The model under review builds one solid part; all positions refer to its coordinate system, in mm. A direction names the side the tool comes from. Coordinates: 2 decimals unless noted, no trailing zeros. Loops run counter-clockwise (first coordinate to the right, second up) from the corner with the lowest first, then second, coordinate; pieces in that order, holes last. Notation, with made-up numbers: M 45,25 L 82,25 A26 cw 82,59 Z; hole C 87.25,-20.5 d7. An arc over 180 degrees is marked long. Use one line per item in the form item = value.
Solid Edge part; units mm, degrees
sketch "Sketch1" plane through (0, 0, 0) normal (0, 0, 1) x (1, 0, 0)
  circle A0 centre (0, 0) radius 7.1374
extrude "Protrusion1" add sketch "Sketch1" along normal blind 6.35
sketch "Sketch2" plane through (0, 0, 0) normal (0, 0, -1) x (0, 1, 0)
  circle A0 centre (0, 0) radius 4.7625
extrude "Protrusion2" add sketch "Sketch2" along normal blind 12.7
sketch "Sketch3" plane through (0, 0, -12.7) normal (0, 0, -1) x (0, 1, 0)
  circle A0 centre (0, 0) radius 3.9688
extrude "Protrusion3" add sketch "Sketch3" along normal blind 12.7
sketch "Sketch4" plane through (0, 0, 6.35) normal (0, 0, 1) x (0, 1, 0)
  line L0 (-2.3876, 1.3131) -> (0, 2.8792)
  line L1 (-2.3876, -1.5424) -> (-2.3876, 1.3131)
  line L2 (-2.3876, -1.5424) -> (0, -2.8792)
  line L3 (2.3876, -1.5424) -> (0, -2.8792)
  line L4 (2.3876, -1.5424) -> (2.3876, 1.3131)
  line L5 (2.3876, 1.3131) -> (0, 2.8792)
extrude "Cutout1" cut sketch "Sketch4" against normal blind 3.175
chamfer "Chamfer1" distance 0.7874 angle 45 1 edges at (0, -3.9688, -25.4)
properties part number "24103079"
1. Machinability: for faces 1 (the face through (0, -3, 6.35)), 2 (the face through (2.2, 1.21, 4.78)), 3 (the face through (2.9, -3.78, -6.26)), which of the approach directions +Z, -Z, +X, -X, +Y, -Y give a long, thin tool a straight path to every point of the face, cutting with its end or side? Answer none if there is none.
Response values:
face_1 = +Z, +X, -X, +Y, -Y
face_2 = +Z
face_3 = -Z
2. Add section B-B (z = -5). State the section outline as (x, y) points (1 decimal).
Response values:
outline = C 0,0 d9.5
3. Add section D-D (z = -16.5). State the section outline as (x, y) points.
Response values:
outline = C 0,0 d7.94
4. Add section C-C (y = -5.25). State the section outline as (x, z) points.
Response values:
outline = M -4.84,0 L 4.84,0 L 4.84,6.35 L -4.84,6.35 Z
5. Insertion check: P1, Ø4, axis at x = 4.5, z = 1, coming from the +Y side; P2, Ø1, axis at x = 5, y = 2, coming from the -Z side; P3, Ø2, axis at y = 3, z = -13, coming from the -X side. Each pin has a flat end and moves straight along its axis. Give the tip position at first contact, or say it passes through.
Response values:
P1 = 6.69
P2 = 0
P3 = -4.3
6. Wall thickness on line 1 along Y through (x, z) = (0.25, -18.5); line 2 along Z through (x, y) = (6.25, 1.25); line 3 along X through (y, z) = (0, -13): over which ranges is each line inside the solid? List them lowest first. Write a range as from..to.
Response values:
line_1 = -3.96..3.96
line_2 = 0..6.35
line_3 = -3.97..3.97
7. The part is to be moulded in two halves that separate along Y. For faces 4 (the face through (2.2, -1.21, 4.78)), 5 (the face through (1.52, 3.666, -18.573)), 6 (the face through (1, -5, 0)), 7 (the face through (0, -2.388, 5)), say which applies: pulls with the +Y half, pulls with the -Y half, needs draft (parallel to the pull), parting line crosses it, or undercut.
Response values:
face_4 = undercut
face_5 = parting line crosses it
face_6 = needs draft
face_7 = undercut
